Geometry: see drawing. Coordinates: mm, zero at the bounding-box minimum. A direction names the side the tool comes from. Give positions to 0.01 mm unless a question says otherwise; leave off trailing zeros. Loops run counter-clockwise (first coordinate to the right, second up) from the corner with the lowest first, then second, coordinate; pieces in that order, holes last. Notation, with made-up numbers: M 7.5,82.25 L 31.5,82.25 A17 cw 31.5,98.25 Z; hole C 64.5,32 d10. An arc over 180 degrees is marked long. Return JSON: item names as keys, results as strings. Group by question number.
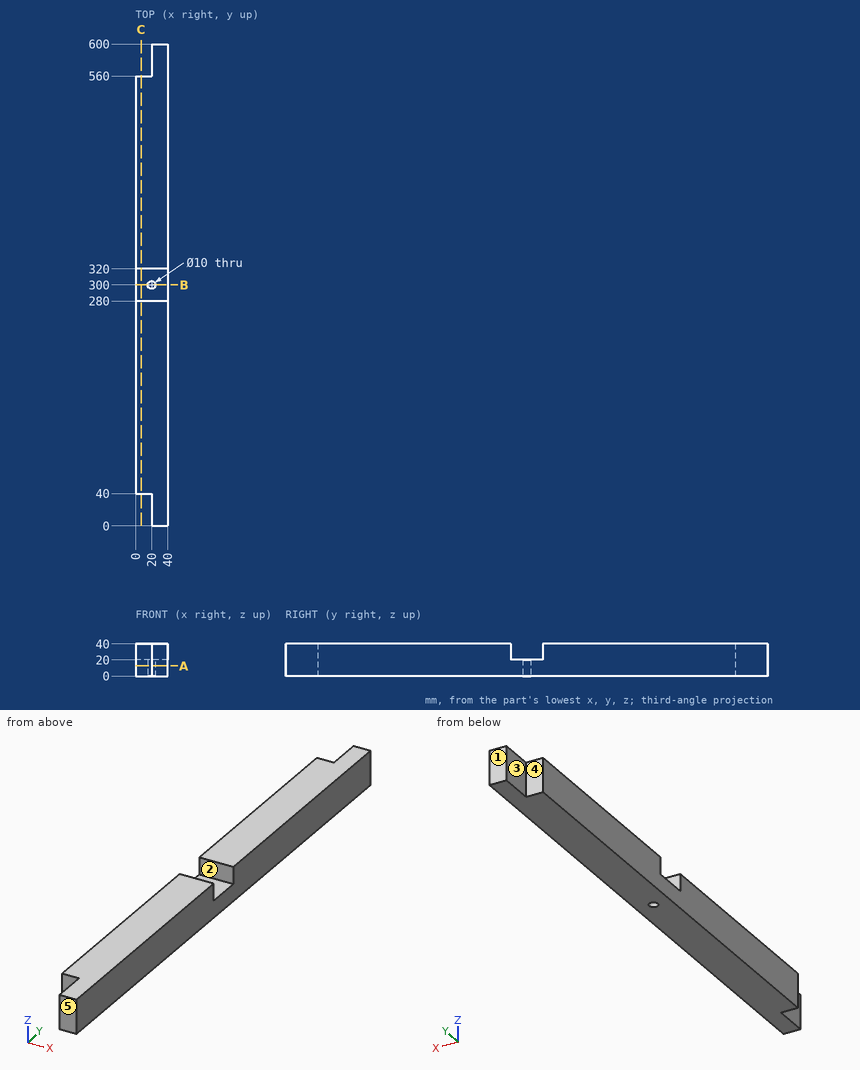
Item 1: Reachability of the marked faces 4 and 5 from +Z, -Z, +X, -X, +Y, -Y: full face, straight path, thin tool, end or side. Return the list, or none.
Item 2: Section A-A, the plane z = 12.5. Return loops of the section in (x, y), then the cut area to 3 significant figures.
Item 3: First-contact query: pin 1 Ø20 at (y, z) = (575.5, 20.5) entering from -X; pin 2 Ø6 at (x, z) = (7.5, 13) entering from -Y; pin 3 Ø6 at (x, z) = (10.5, 19) entering from +Y. Flat tips, straight axial feed; report the tip coordinate or a pass-through.
Item 4: Section B-B, the plane y = 300. Return loops of the section in (x, z), then the cut area to 3 significant figures.
Item 5: Pull-direction query (Y, two-part tool) for the marked faces 1, 2 and 3; classes: pulls with the +Y half, pulls with the -Y half, needs draft (parallel to the pull), parting line crosses it, or undercut.
Item 6: Section C-C, the plane x = 7. Return loops of the section in (y, z).
Item 7: Material intervals for line 1 (X direction, y = 300, z = 9); line 2 (Y direction, x = 33.5, z = 30.5); line 3 (Y direction, x = 8.5, z = 27), sorted ascending. Write a range as from..to.
Answer below:
{
 "1": {"face 4": "+Z, -Z, -X, +Y", "face 5": "+Z, -Z, +X, -X, -Y"},
 "2": {"outline": "M 0,40 L 20,40 L 20,0 L 40,0 L 40,600 L 20,600 L 20,560 L 0,560 Z; hole C 20,300 d10", "area": "22,300 mm^2"},
 "3": {"pin 1": "x = 20", "pin 2": "y = 40", "pin 3": "y = 560"},
 "4": {"outline": "M 0,0 L 15,0 L 15,20 L 0,20 Z; M 25,0 L 40,0 L 40,20 L 25,20 Z", "area": "600 mm^2"},
 "5": {"face 1": "pulls with the +Y half", "face 2": "undercut", "face 3": "needs draft"},
 "6": {"outline": "M 40,0 L 560,0 L 560,40 L 320,40 L 320,20 L 280,20 L 280,40 L 40,40 Z"},
 "7": {"line 1": "0..15, 25..40", "line 2": "0..280, 320..600", "line 3": "40..280, 320..560"}
}
